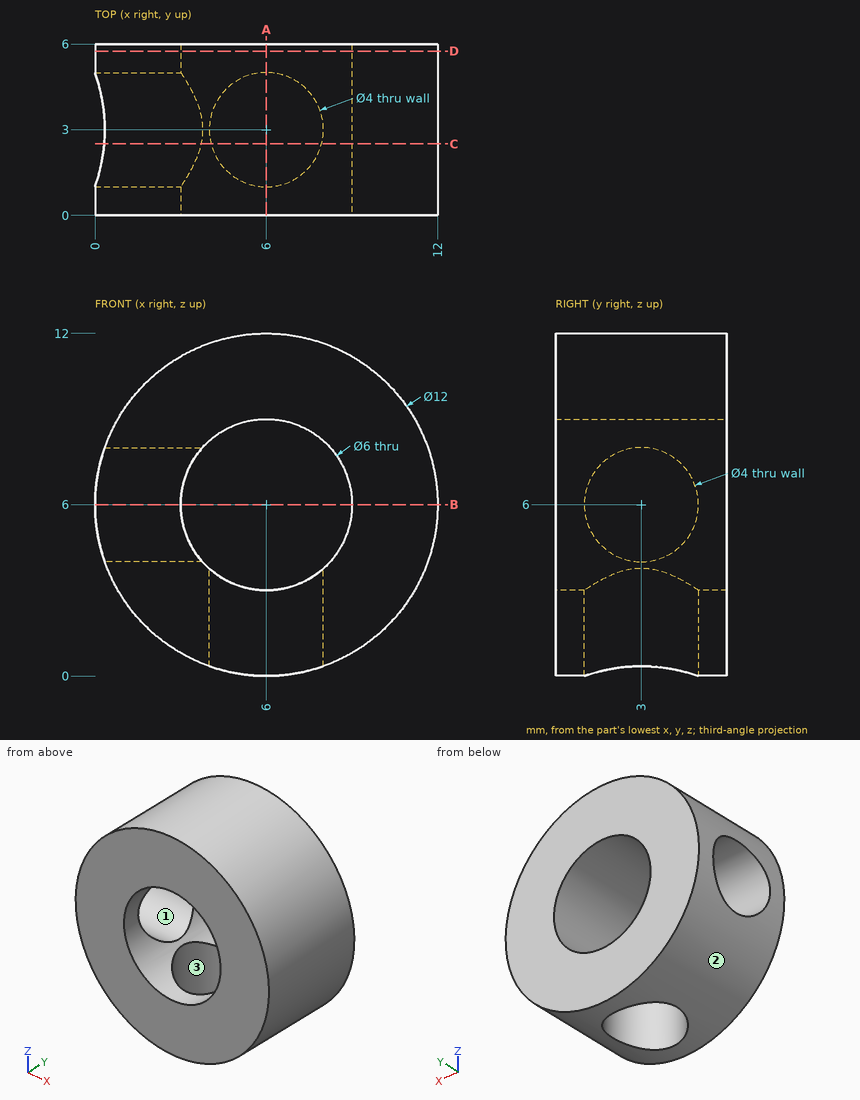
Here's the drawing with two shaded views (mm, measured from the low corner). I have some questions. Coordinates: 2 decimals unless noted, no trailing zeros. Loops run counter-clockwise (first coordinate to the right, second up) from the corner with the lowest first, then second, coordinate; pieces in that order, holes last. Notation, with made-up numbers: (68.25, -12.75) -> (111.25, -12.75) arc R19 ccw to (111.25, 10.25) -> close; hole circle Ø1 at (-21.5, 29.25). An arc over 180 degrees is marked (long way). Answer as a JSON object with one key per item and string values.
1) Imagine slicing it at D-D (y = 5.75). Please give me the cut outline in (x, z), then the cut area to 3 significant figures.
Results:
{"outline": "circle Ø12 at (6, 6); hole circle Ø6 at (6, 6)", "area": "84.8 mm^2"}
2) For P1, Ø1, axis at x = 2.5, y = 3.5, coming from the -Z side; P2, Ø2, axis at x = 11, y = 5, coming from the -Z side; P3, Ø2, axis at x = 9, y = 2, coming from the -Z side, each with a flat end and sliding along its axis, tell me the tip position at first contact or that it passes through.
Results:
{"P1": "stops at z = 0.8", "P2": "stops at z = 1.53", "P3": "stops at z = 0.34"}
3) Imagine slicing it at A-A (x = 6). Please give me the cut outline in (y, z), then the cut area to 3 significant figures.
Results:
{"outline": "(0, 0) -> (1, 0) -> (1, 3) -> (0, 3) -> close; (0, 9) -> (6, 9) -> (6, 12) -> (0, 12) -> close; (5, 0) -> (6, 0) -> (6, 3) -> (5, 3) -> close", "area": "24.0 mm^2"}
4) If I drill on line 1 (Y direction, x = 1.05, z = 6); line 2 (X direction, y = 5.5, z = 6); line 3 (Z direction, x = 8.25, y = 5), over which ranges is the centre line in solid material (lowest first)?
Results:
{"line 1": "y = 0 to 1, 5 to 6", "line 2": "x = 0 to 3, 9 to 12", "line 3": "z = 0.44 to 4.02, 7.98 to 11.56"}
5) Imagine slicing it at B-B (z = 6). Please give me the cut outline in (x, y), then the cut area to 3 significant figures.
Results:
{"outline": "(0, 0) -> (3, 0) -> (3, 1) -> (0, 1) -> close; (0, 5) -> (3, 5) -> (3, 6) -> (0, 6) -> close; (9, 0) -> (12, 0) -> (12, 6) -> (9, 6) -> close", "area": "24.0 mm^2"}
6) Thinking about a two-plate mould opening in X: for the marked faces 1, 2 and 3, which applies, pulls with the +X half, pulls with the -X half, needs draft (parallel to the pull), parting line crosses it, or undercut?
Results:
{"face 1": "needs draft", "face 2": "parting line crosses it", "face 3": "undercut"}
7) Imagine slicing it at C-C (y = 2.5). Please give me the cut outline in (x, z), then the cut area to 3 significant figures.
Results:
{"outline": "(0.32, 4.06) arc R6 ccw to (4.06, 0.32) -> (4.06, 3.71) arc R3 cw to (3.71, 4.06) -> close; (0.32, 7.94) -> (3.71, 7.94) arc R3 cw (long way) to (7.94, 3.71) -> (7.94, 0.32) arc R6 ccw (long way) to start", "area": "60.7 mm^2"}
